The figure shows three views and two pictorial views of one solid part (mm, origin at its lowest corner). Answer the questions. Give positions to 0.01 mm unless a question says otherwise; leave off trailing zeros. Write each loop counter-clockwise with the first axis right and the second up, starting at its lowest first coordinate (ties: lowest second). Pieces come first, ordered by that corner, then holes. Notation, with made-up numbers: (-27, 42) -> (-20, 42) arc R20 ccw to (-20, 54) -> close; hole circle Ø11 at (5.25, 25). An arc over 180 degrees is marked (long way). Write each question's results on one line, items separated by ' | '. Start each with the question number.
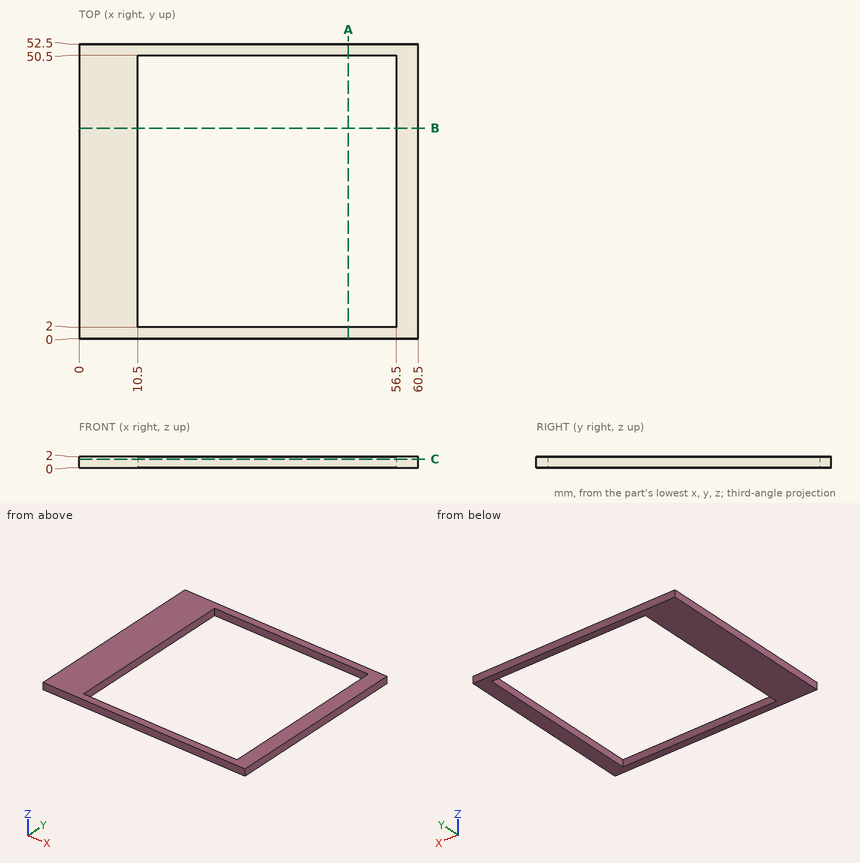
1. Section A-A (x = 48) is taken. Write down the section's boundary in (y, z).
2. Consider probe 1 along Y at (x, z) = (46.5, 1.6); probe 2 along X at (y, z) = (42.5, 0.3). Determine where each line is inside the solid, lowest interval first. Write a range as [from, to].
3. Section C-C (z = 1.55) is taken. Write down the section's boundary in (x, y).
4. Section B-B (y = 37.5) is taken. Write down the section's boundary in (x, z).
Results:
1) outline: (0, 0) -> (2, 0) -> (2, 2) -> (0, 2) -> close; (50.5, 0) -> (52.5, 0) -> (52.5, 2) -> (50.5, 2) -> close
2) probe 1: y = [0, 2], [50.5, 52.5] | probe 2: x = [0, 10.5], [56.5, 60.5]
3) outline: (0, 0) -> (60.5, 0) -> (60.5, 52.5) -> (0, 52.5) -> close; hole (10.5, 2) -> (56.5, 2) -> (56.5, 50.5) -> (10.5, 50.5) -> close
4) outline: (0, 0) -> (10.5, 0) -> (10.5, 2) -> (0, 2) -> close; (56.5, 0) -> (60.5, 0) -> (60.5, 2) -> (56.5, 2) -> close
